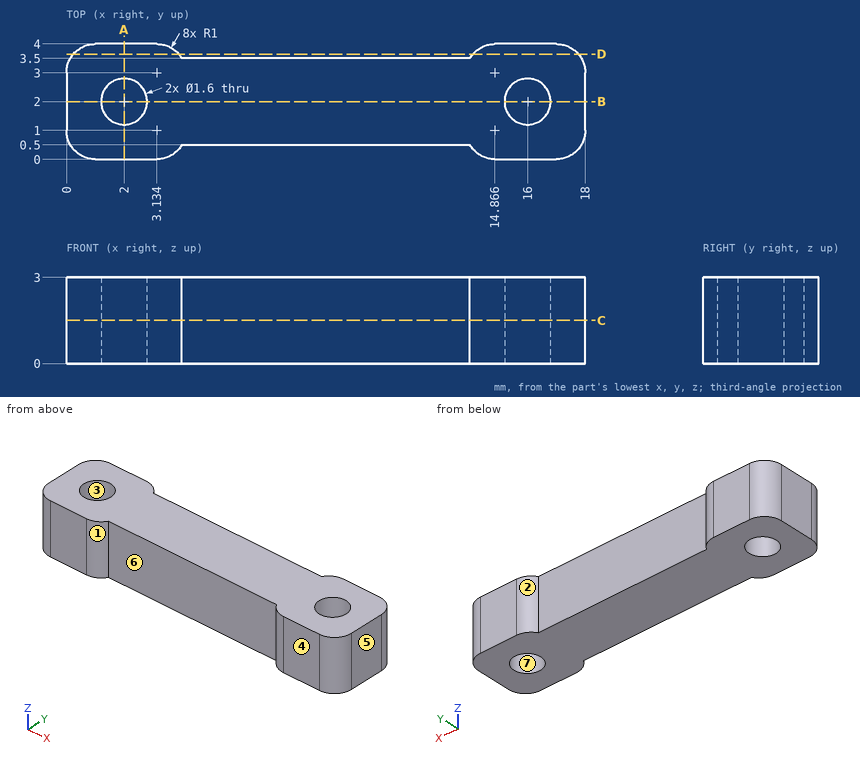
Verification items for this drawing (mm, ordinates from the low corner). A direction names the side the tool comes from. Give positions to 0.01 mm unless a question says otherwise; leave off trailing zeros. Write each loop counter-clockwise with the first axis right and the second up, starting at its lowest first coordinate (ties: lowest second). Pieces come first, ordered by that corner, then holes. Notation, with made-up numbers: (47.5, 19.25) -> (103.5, 19.25) arc R11 ccw to (103.5, 34.25) -> close; hole circle Ø2 at (-18, 12.25). An arc over 180 degrees is marked (long way). Use CSV: the item, a comma, the result in double quotes. Start each with the question number.
Q1. Tool access check on the marked faces 1, 2 and 3. Record the directions out of +Z, -Z, +X, -X, +Y, -Y that give a thin tool (end or side, any length) a straight path to the whole face; none if there is none.
Q2. Scan lines: line 1 along Y through (x, z) = (16, 0.8); line 2 along X through (y, z) = (1.6, 2.05); line 3 along X through (y, z) = (1.4, 2). Record each from-to range of solid material in increasing order.
Q3. Cross-section at C-C on z = 1.5. Enter the section's corners in (x, y), and give its area (3 significant figures).
Q4. Cross-section at D-D on y = 3.65. Enter the section's corners in (x, z).
Q5. Cross-section at A-A on x = 2. Enter the section's corners in (y, z), and give its area (3 significant figures).
Q6. Cross-section at B-B on y = 2. Enter the section's corners in (x, z).
Q7. Release check for a two-part mould opening along X. For the marked faces 4, 5, 6 and 7 record: +X half, -X half, draft (parallel to the pull), parting line (faces both ways), or undercut.
Q8. Depth check by flat-ended pin: P1, Ø1, axis at x = 8.5, z = 1, coming from the -Y side; P2, Ø1.5, axis at x = 14, z = 0.5, coming from the -Y side. Enter the tip coordinate at first touch or a pass-through.
Working result:
1,face 1,"+Z, -Z, -Y"
1,face 2,"+Z, -Z, +Y"
1,face 3,"+Z, -Z"
2,line 1,"y = 0 to 1.2, 2.8 to 4"
2,line 2,"x = 0 to 1.31, 2.69 to 15.31, 16.69 to 18"
2,line 3,"x = 0 to 1.47, 2.53 to 15.47, 16.53 to 18"
3,outline,"(0, 1) arc R1 ccw to (1, 0) -> (3.13, 0) arc R1 ccw to (4, 0.5) -> (14, 0.5) arc R1 ccw to (14.87, 0) -> (17, 0) arc R1 ccw to (18, 1) -> (18, 3) arc R1 ccw to (17, 4) -> (14.87, 4) arc R1 ccw to (14, 3.5) -> (4, 3.5) arc R1 ccw to (3.13, 4) -> (1, 4) arc R1 ccw to (0, 3) -> close; hole circle Ø1.6 at (2, 2); hole circle Ø1.6 at (16, 2)"
3,area,"56.6 mm^2"
4,outline,"(0.24, 0) -> (3.89, 0) -> (3.89, 3) -> (0.24, 3) -> close; (14.11, 0) -> (17.76, 0) -> (17.76, 3) -> (14.11, 3) -> close"
5,outline,"(0, 0) -> (1.2, 0) -> (1.2, 3) -> (0, 3) -> close; (2.8, 0) -> (4, 0) -> (4, 3) -> (2.8, 3) -> close"
5,area,"7.20 mm^2"
6,outline,"(0, 0) -> (1.2, 0) -> (1.2, 3) -> (0, 3) -> close; (2.8, 0) -> (15.2, 0) -> (15.2, 3) -> (2.8, 3) -> close; (16.8, 0) -> (18, 0) -> (18, 3) -> (16.8, 3) -> close"
7,face 4,"draft"
7,face 5,"+X half"
7,face 6,"undercut"
7,face 7,"undercut"
8,P1,"stops at y = 0.5"
8,P2,"stops at y = 0.01"
